Design review of the part built by this model. Coordinates are the model's own, in mm. Coordinates: 2 decimals unless noted, no trailing zeros. Write each loop counter-clockwise with the first axis right and the second up, starting at its lowest first coordinate (ties: lowest second). Pieces come first, ordered by that corner, then holes.
Q1. Clearance check with flat-ended pins moving along their axes: pin 1 Ø10 at (y, z) = (-30.5, 21) entering from -X; pin 2 Ø3 at (y, z) = (44.5, 22) entering from +X; pin 3 Ø1 at (y, z) = (-54.5, 28) entering from +X. State where each tip first meets the part, or that it passes through.
Q2. Add section B-B, the plane x = 165.5. Give the boundary of the cut face in (y, z).
Q3. Add section D-D, the plane x = 17. Give the boundary of the cut face in (y, z).
Q4. Add section A-A, the plane y = -69.5. Give the boundary of the cut face in (x, z).
Q5. The part is to be moulded in two halves that separate along X. For faces 1 (the face through (-190, -1, 5)), 2 (the face through (165, 1, 10)), 3 (the face through (164.701, 1.4, 25.717)), 4 (the face through (-3, 1, 0)), say which applies: +X half, -X half, draft (parallel to the pull), parting line (faces both ways), or undercut.
Q6. Add section C-C, the plane z = 20.5. Give the boundary of the cut face in (x, y).
Q7. To check wall thickness, follow probe 1 along X at (y, z) = (81, 18); probe 2 along Z at (x, y) = (-163.5, 18); probe 3 along X at (y, z) = (66, 23.5). State the ranges of each line that lie inside material, in increasing order.
from build123d import *

# Parameters (mm, degrees)
SKETCH1_W                       = 380
SKETCH1_H                       = 200
FOOT_DEPTH                      = 10
BOSS_EXTRUDE2_REACH             = 216.942
SKETCH2_R                       = 15.273641531
SKETCH2_R_2                     = 8.942985805
BOSS_EXTRUDE2_DIRECTION_2_REACH = 216.942


with BuildPart() as part:
    # Sketch1 → Foot (new body)
    with BuildSketch(Plane.XY):
        Rectangle(SKETCH1_W, SKETCH1_H)
    extrude(amount=FOOT_DEPTH)

    # Boss-Extrude2: up to this face of the body (flat: up to its plane)
    boss_extrude2_end = Plane(part.part.faces().sort_by_distance((0, 100, 5))[0])
    # Sketch2 → Boss-Extrude2 (add, up to the picked face)
    with BuildSketch(Plane(origin=(0, 0, 0), x_dir=(1, 0, 0), z_dir=(0, 1, 0)), mode=Mode.PRIVATE) as boss_extrude2_sk1:
        with Locations((165.004857041, -16.778784358)):
            Circle(SKETCH2_R)
        with Locations((165.004857041, -16.778784358)):
            Circle(SKETCH2_R_2, mode=Mode.SUBTRACT)
    boss_extrude2_tool1 = split(extrude(boss_extrude2_sk1.sketch, amount=BOSS_EXTRUDE2_REACH, mode=Mode.PRIVATE), bisect_by=boss_extrude2_end, keep=Keep.BOTH, mode=Mode.PRIVATE)
    add(boss_extrude2_tool1.solids().sort_by(Axis((150.163219, 0, 16.778784), (0, 1, 0)))[0])

    # Boss-Extrude2 direction 2: up to this face of the body (flat: up to its plane)
    boss_extrude2_direction_2_end = Plane(part.part.faces().sort_by_distance((0, -100, 5))[0])
    # Sketch2 → Boss-Extrude2 direction 2 (add, up to the picked face)
    with BuildSketch(Plane(origin=(0, 0, 0), x_dir=(1, 0, 0), z_dir=(0, 1, 0)), mode=Mode.PRIVATE) as boss_extrude2_direction_2_sk1:
        with Locations((165.004857041, -16.778784358)):
            Circle(SKETCH2_R)
        with Locations((165.004857041, -16.778784358)):
            Circle(SKETCH2_R_2, mode=Mode.SUBTRACT)
    boss_extrude2_direction_2_tool1 = split(extrude(boss_extrude2_direction_2_sk1.sketch, amount=-BOSS_EXTRUDE2_DIRECTION_2_REACH, mode=Mode.PRIVATE), bisect_by=boss_extrude2_direction_2_end, keep=Keep.BOTH, mode=Mode.PRIVATE)
    add(boss_extrude2_direction_2_tool1.solids().sort_by(Axis((150.163219, 0, 16.778784), (0, -1, 0)))[0])


solid = part.part
Here are the results:
1. pin 1: stops at x = 149.73
1. pin 2: stops at x = 179.82
1. pin 3: stops at x = 175.88
2. outline: (-100, 0) - (100, 0) - (100, 10) - (-100, 10) - close; (-100, 25.71) - (100, 25.71) - (100, 32.04) - (-100, 32.04) - close
3. outline: (-100, 0) - (100, 0) - (100, 10) - (-100, 10) - close
4. outline: (-190, 0) - (190, 0) - (190, 10) - (178.69, 10) arc R15.27 ccw (long way) to (151.32, 10) - (-190, 10) - close; hole (159.17, 10) - (170.84, 10) arc R8.94 ccw (long way) to start
5. face 1: -X half
5. face 2: undercut
5. face 3: undercut
5. face 4: draft
6. outline: (150.19, -100) - (156.87, -100) - (156.87, 100) - (150.19, 100) - close; (173.14, -100) - (179.82, -100) - (179.82, 100) - (173.14, 100) - close
7. probe 1: x = 149.78 to 156.15, 173.86 to 180.23
7. probe 2: z = 0 to 10
7. probe 3: x = 151.29 to 159.11, 170.9 to 178.72
